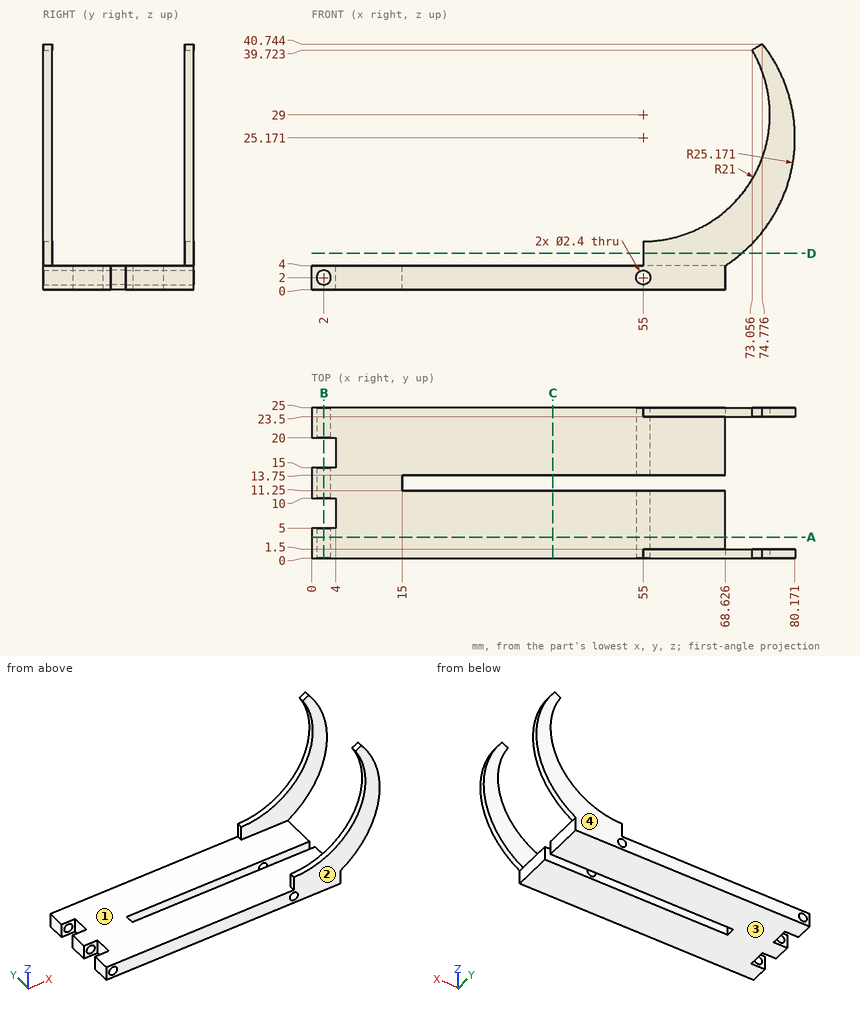
Could you check a few things on this drawing? It's one solid part, dimensions in mm from its lowest x, y, z. Round coordinates to 2 decimals unless told otherwise and drop trailing zeros. Loops run counter-clockwise (first coordinate to the right, second up) from the corner with the lowest first, then second, coordinate; pieces in that order, holes last. Notation, with made-up numbers: M 85.5,36.25 L 126.5,36.25 A26 ccw 126.5,51.25 Z; hole C 85.25,-10 d11. An arc over 180 degrees is marked long. Write item = value, one per line. Start each with the question number.
(1) Suppose I cut it at C-C on x = 40. Write out the boundary of the cut face in (y, z).
(2) I'm going to push flat-ended pins straight in: P1, Ø1.4, axis at x = 2, z = 2, coming from the +Y side; P2, Ø0.8, axis at y = 12.5, z = 2, coming from the +X side; P3, Ø7.5, axis at x = 37.5, y = 15, coming from the +Z side; P4, Ø3, axis at y = 20.5, z = 2, coming from the +X side. Where does each tip first touch, or does it pass through?
(3) If we mould it in two halves opening along Y, with no side actions, what happens to the marked faces 1, 2, 3 and 4? For each: released by +Y, released by -Y, zero draft, split by the parting line, or undercut.
(4) Suppose I cut it at B-B on x = 2. Write out the boundary of the cut face in (y, z).
(5) Suppose I cut it at D-D on z = 6. Write out the boundary of the cut face in (x, y).
(6) I need wall thicknesses on line 1 along Z through (x, y) = (55, 17); line 2 along Y through (x, z) = (20, 2.5); line 3 along Z through (x, y) = (6, 16.75). Which ranges of each line are inside material? Lowest first, please.
(7) Suppose I cut it at A-A on y = 3.5. Write out the boundary of the cut face in (x, z).
Answer block:
q1.outline = M 0,0 L 11.25,0 L 11.25,4 L 0,4 Z; M 13.75,0 L 25,0 L 25,4 L 13.75,4 Z
q2.P1 = through
q2.P2 = 15
q2.P3 = 4
q2.P4 = 68.63
q3.face_1 = undercut
q3.face_2 = released by -Y
q3.face_3 = zero draft
q3.face_4 = released by +Y
q4.outline = M 0,0 L 5,0 L 5,0.8 L 0,0.8 Z; M 0,3.2 L 5,3.2 L 5,4 L 0,4 Z; M 10,0 L 15,0 L 15,0.8 L 10,0.8 Z; M 10,3.2 L 15,3.2 L 15,4 L 10,4 Z; M 20,0 L 25,0 L 25,0.8 L 20,0.8 Z; M 20,3.2 L 25,3.2 L 25,4 L 20,4 Z
q5.outline = M 55,0 L 71.31,0 L 71.31,1.5 L 55,1.5 Z; M 55,23.5 L 71.31,23.5 L 71.31,25 L 55,25 Z
q6.line_1 = 0 to 0.8, 3.2 to 4
q6.line_2 = 0 to 11.25, 13.75 to 25
q6.line_3 = 0 to 4
q7.outline = M 0,0 L 68.63,0 L 68.63,4 L 0,4 Z; hole C 2,2 d2.4; hole C 55,2 d2.4
